from build123d import *

# Parameters (mm, degrees)
SKETCH7_R           = 1.5875
BOSS_EXTRUDE2_DEPTH = 3.175
SKETCH5_R           = 6.35
CUT_EXTRUDE1_DEPTH  = 41.348883888
SKETCH8_R           = 6.35
EXTRUDE1_DEPTH      = 57.15
CUT_EXTRUDE2_DEPTH  = 12.7
SKETCH10_R          = 4.7625
EXTRUDE2_DEPTH      = 30


with BuildPart() as part:
    # Sketch4 → Boss-Revolve2 (revolve)
    with BuildSketch(Plane.XY):
        Polygon((-47.625, 0), (-47.625, -6.35), (-34.925, -6.35), (-34.925, -9.525), (28.575, -9.525), (28.575, 0), align=None)
    revolve(axis=Axis((-47.625, 0, 0), (1, 0, 0)))

    # Sketch7 → Boss-Extrude2 (add)
    with BuildSketch(Plane(origin=(28.575, 29.318732004, 10.174246846), x_dir=(0, 0.707106781, -0.707106781), z_dir=(1, 0, 0))):
        with BuildLine():
            Line((-20.873950462, -12.811868036), (-10.250193405, -15.65849516))
            ThreePointArc((-10.250193405, -15.65849516), (-4.556939156, -18.945497033), (-1.269937284, -24.638751281))
            Line((-1.269937284, -24.638751281), (1.57668984, -35.262508339))
            ThreePointArc((1.57668984, -35.262508339), (-0.066811096, -41.396137336), (-6.200440093, -43.039638272))
            Line((-6.200440093, -43.039638272), (-16.82419715, -40.193011148))
            ThreePointArc((-16.82419715, -40.193011148), (-22.517451399, -36.906009275), (-25.804453271, -31.212755027))
            Line((-25.804453271, -31.212755027), (-28.651080396, -20.588997969))
            ThreePointArc((-28.651080396, -20.588997969), (-27.007579459, -14.455368972), (-20.873950462, -12.811868036))
        make_face()
        with Locations((-22.517451399, -18.945497033)):
            Circle(SKETCH7_R, mode=Mode.SUBTRACT)
        with Locations((-4.556939156, -36.906009275)):
            Circle(SKETCH7_R, mode=Mode.SUBTRACT)
    extrude(amount=-BOSS_EXTRUDE2_DEPTH)

    # Sketch5 → Cut-Extrude1 (cut)
    with BuildSketch(Plane(origin=(28.575, 0, 0), x_dir=(0, 0, -1), z_dir=(1, 0, 0))):
        Circle(SKETCH5_R)
    extrude(amount=-CUT_EXTRUDE1_DEPTH, mode=Mode.SUBTRACT)

    # Sketch8 → Extrude1 (add)
    with BuildSketch(Plane(origin=(-12.773883888, 0, 0), x_dir=(0, 0, -1), z_dir=(1, 0, 0))):
        Circle(SKETCH8_R)
    extrude(amount=EXTRUDE1_DEPTH)

    # Sketch9 → Cut-Extrude2 (cut)
    with BuildSketch(Plane(origin=(44.376116112, 0, 0), x_dir=(0, 0, -1), z_dir=(1, 0, 0))):
        with BuildLine():
            Line((-6.148361062, 1.5875), (6.148361062, 1.5875))
            ThreePointArc((6.148361062, 1.5875), (0, 6.35), (-6.148361062, 1.5875))
        make_face()
    extrude(amount=-CUT_EXTRUDE2_DEPTH, mode=Mode.SUBTRACT)

    # Sketch10 → Extrude2 (add)
    with BuildSketch(Plane(origin=(0, 0, 0), x_dir=(1, 0, 0), z_dir=(0, 1, 0))):
        with Locations((-22.225, 0)):
            Circle(SKETCH10_R)
    extrude(amount=EXTRUDE2_DEPTH)


solid = part.part
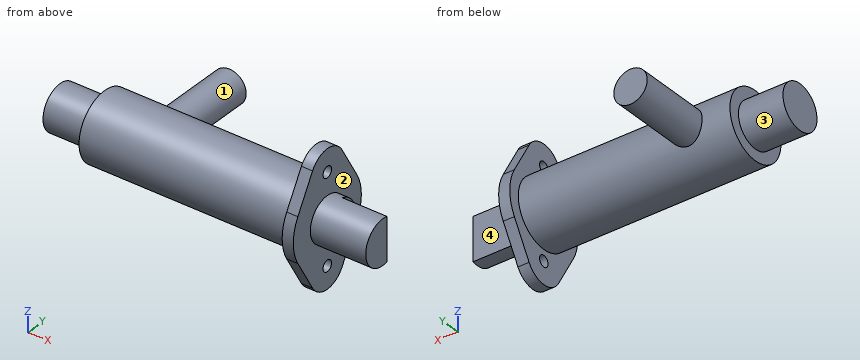
The listing builds one solid part. Answer for the finished solid, in the listing's coordinates (mm). Face numbers are marked on the shaded views. A direction names the side the tool comes from. Coordinates: 2 decimals unless noted, no trailing zeros. Write each loop counter-clockwise with the first axis right and the second up, starting at its lowest first coordinate (ties: lowest second). Pieces come first, ordered by that corner, then holes. Notation, with made-up numbers: M 66,22.5 L 92,22.5 A22 ccw 92,36.5 Z; hole C -15.5,2 d10. An arc over 180 degrees is marked long. Use one line per item in the form item = value.
Item 1: For the marked faces 1, 2, 3 and 4, determine the directions among +Z, -Z, +X, -X, +Y, -Y from which every point of the face is accessible in a straight line to the end or side of a thin tool.
Model answer:
face_1 = +Y
face_2 = +X
face_3 = -X
face_4 = +Z, -Z, +X, +Y
Item 2: Find section C-C, the plane x = -37. Give the vertices of the cut face in (y, z), plus the area to 3 significant figures.
Model answer:
outline = C 0,0 d12.7
area = 127 mm2
Item 3: Find section A-A, the plane z = 12.7. Give the vertices of the cut face in (x, y) (1 decimal), plus the area to 3 significant figures.
Model answer:
outline = M 25.4,-7.3 L 28.6,-7.3 L 28.6,-1.6 L 25.4,-1.6 Z; M 25.4,1.6 L 28.6,1.6 L 28.6,7.3 L 25.4,7.3 Z
area = 36.5 mm2
Item 4: Find section D-D, the plane y = 3. Give the vertices of the cut face in (x, z) (3 decimals), plus the area to 3 significant figures.
Model answer:
outline = M -47.625,-5.597 L -34.925,-5.597 L -34.925,-9.04 L 25.4,-9.04 L 25.4,-18.297 L 28.575,-18.297 L 28.575,-5.597 L 31.676,-5.597 L 31.676,5.597 L 28.575,5.597 L 28.575,18.297 L 25.4,18.297 L 25.4,9.04 L -34.925,9.04 L -34.925,5.597 L -47.625,5.597 Z
area = 1,380 mm2
Item 5: Find the intervals of material crossed by probe 1 along X at (y, z) = (2, 6.5) (3 decimals); probe 2 along X at (y, z) = (2, 1.5) (3 decimals); probe 3 along Y at (x, z) = (27.7, -12.7), in increasing order.
Model answer:
probe_1 = -34.925 to 28.575
probe_2 = -47.625 to 31.676
probe_3 = -7.33 to -1.59, 1.59 to 7.33
Item 6: Given P1, Ø1.5, axis at x = 26.5, z = 6, coming from the +Y side; P2, Ø1.5, axis at y = -3, z = 9, coming from the +X side (3 decimals); P3, Ø1.5, axis at x = 9, z = -9.5, coming from the +Y side, each flat-ended and moving along its own axis, determine where each tip first touches the part or whether it passes through.
Model answer:
P1 = 11.56
P2 = 28.575
P3 = 3.76
